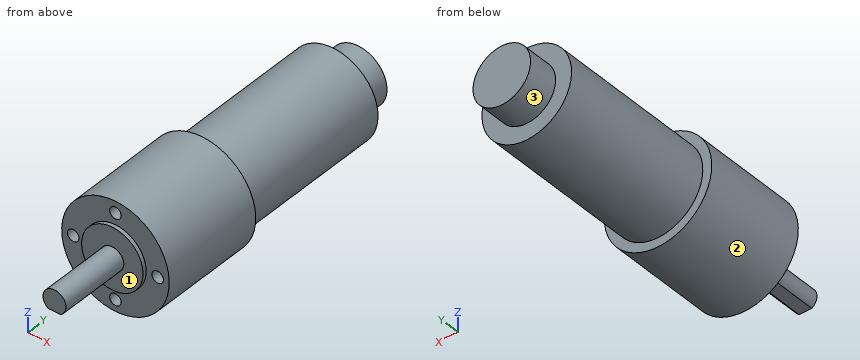
from build123d import *

# Parameters (mm, degrees)
SKETCH_1_R          = 14
EXTRUDE_1_DEPTH     = 27.7
SKETCH_3_R          = 11.669632126
EXTRUDE_2_DEPTH     = 42
SKETCH_8_R          = 7.5
EXTRUDE_4_DEPTH     = 8
SKETCH_9_R          = 8
EXTRUDE_5_DEPTH     = 1
SKETCH_5_R          = 3
EXTRUDE_3_DEPTH     = 18.5
CUT_EXTRUDE_START   = -12
CUT_EXTRUDE_2_DEPTH = 12
SKETCH_4_R          = 1.5
CUT_EXTRUDE_1_DEPTH = 4


with BuildPart() as part:
    # 草图1 → 凸台-拉伸1 (new body)
    with BuildSketch(Plane(origin=(0, 0, 0), x_dir=(1, 0, 0), z_dir=(0, 1, 0))):
        with Locations(Location((0, 0, 0), (0, 0, 270))):
            Circle(SKETCH_1_R)
    extrude(amount=EXTRUDE_1_DEPTH)

    # 草图3 → 凸台-拉伸2 (add)
    with BuildSketch(Plane(origin=(0, 27.7, 0), x_dir=(1, 0, 0), z_dir=(0, 1, 0))):
        with Locations(Location((0, 0, 0), (0, 0, 90))):
            Circle(SKETCH_3_R)
    extrude(amount=EXTRUDE_2_DEPTH)

    # 草图8 → 凸台-拉伸4 (add)
    with BuildSketch(Plane(origin=(0, 69.7, 0), x_dir=(1, 0, 0), z_dir=(0, 1, 0))):
        with Locations(Location((0, 0, 0), (0, 0, 270))):
            Circle(SKETCH_8_R)
    extrude(amount=EXTRUDE_4_DEPTH)

    # 草图9 → 凸台-拉伸5 (add)
    with BuildSketch(Plane.XZ):
        with Locations(Location((0, 0, 0), (0, 0, 90))):
            Circle(SKETCH_9_R)
    extrude(amount=EXTRUDE_5_DEPTH)

    # 草图5 → 凸台-拉伸3 (add)
    with BuildSketch(Plane.XZ.offset(1)):
        with Locations(Location((0, 0, 0), (0, 0, 270))):
            Circle(SKETCH_5_R)
    extrude(amount=EXTRUDE_3_DEPTH)

    # 草图7 → 切除-拉伸2 (cut)
    with BuildSketch(Plane.XZ.offset(19.5).offset(CUT_EXTRUDE_START)):
        with BuildLine():
            Line((-1.658312395, -2.5), (1.658312395, -2.5))
            ThreePointArc((1.658312395, -2.5), (0, -3), (-1.658312395, -2.5))
        make_face()
    extrude(amount=CUT_EXTRUDE_2_DEPTH, mode=Mode.SUBTRACT)

    # 草图4 → 切除-拉伸1 (cut)
    with BuildSketch(Plane.XZ):
        with Locations(Location((0, 11, 0), (0, 0, 270))):
            Circle(SKETCH_4_R)
        with Locations(Location((11, 0, 0), (0, 0, 270))):
            Circle(SKETCH_4_R)
        with Locations(Location((0, -11, 0), (0, 0, 270))):
            Circle(SKETCH_4_R)
        with Locations(Location((-11, 0, 0), (0, 0, 270))):
            Circle(SKETCH_4_R)
    extrude(amount=-CUT_EXTRUDE_1_DEPTH, mode=Mode.SUBTRACT)


solid = part.part
Verification items for the finished model (mm, model axes). Face numbers are marked on the shaded views. A direction names the side the tool comes from. Give positions to 0.01 mm unless a question says otherwise; leave off trailing zeros. Order: outer loops, then holes, each group sorted by start corner. A loop starts at its lowest first (then second) coordinate and runs counter-clockwise, first axis right, second up. Notation, with made-up numbers: (31, 26.25) -> (77, 26.25) arc R19 ccw to (77, 63.25) -> close; hole circle Ø11 at (78.25, 23). An arc over 180 degrees is marked (long way). Answer as CSV lines item,"result".
Q1. Sectioned sample at C-C on y = 15. Record the cut outline in (x, z).
Solutions:
outline,"circle Ø28 at (0, 0)"
Q2. Sectioned sample at A-A on z = 0. Record the cut outline in (x, y).
Solutions:
outline,"(-14, 0) -> (-12.5, 0) -> (-12.5, 4) -> (-9.5, 4) -> (-9.5, 0) -> (-8, 0) -> (-8, -1) -> (-3, -1) -> (-3, -19.5) -> (3, -19.5) -> (3, -1) -> (8, -1) -> (8, 0) -> (9.5, 0) -> (9.5, 4) -> (12.5, 4) -> (12.5, 0) -> (14, 0) -> (14, 27.7) -> (11.67, 27.7) -> (11.67, 69.7) -> (7.5, 69.7) -> (7.5, 77.7) -> (-7.5, 77.7) -> (-7.5, 69.7) -> (-11.67, 69.7) -> (-11.67, 27.7) -> (-14, 27.7) -> close"
Q3. Depth check by flat-ended pin: pin 1 (1.7 mm diameter, centred on x = -0.5, y = -14, fed in from -Z); pin 2 (2.5 mm diameter, centred on x = 10.5, z = 0.5, fed in from -Y); pin 3 (5 mm diameter, centred on y = 44, z = 10.5, fed in from +X). Enter the tip coordinate at first touch or a pass-through.
Solutions:
pin 1,"stops at z = -2.5"
pin 2,"stops at y = 0"
pin 3,"stops at x = 8.5"
Q4. Scan lines: probe 1 along X at (y, z) = (2.9, 0); probe 2 along X at (y, z) = (20, -0.25); probe 3 along X at (y, z) = (0.5, -12.25). Record each from-to range of solid material in increasing order.
Solutions:
probe 1,"x = -14 to -12.5, -9.5 to 9.5, 12.5 to 14"
probe 2,"x = -14 to 14"
probe 3,"x = -6.78 to -0.83, 0.83 to 6.78"
Q5. Access from +Z, -Z, +X, -X, +Y, -Y to the whole of each face (thin tool, end or side, straight path). Record for the marked faces 1, 2 and 3.
Solutions:
face 1,"-Y"
face 2,"+Y, -Y"
face 3,"+Y"
Q6. Sectioned sample at D-D on z = -4.75. Record the cut outline in (x, y), plus the area to 3 significant figures.
Solutions:
outline,"(-13.17, 0) -> (-6.44, 0) -> (-6.44, -1) -> (6.44, -1) -> (6.44, 0) -> (13.17, 0) -> (13.17, 27.7) -> (10.66, 27.7) -> (10.66, 69.7) -> (5.8, 69.7) -> (5.8, 77.7) -> (-5.8, 77.7) -> (-5.8, 69.7) -> (-10.66, 69.7) -> (-10.66, 27.7) -> (-13.17, 27.7) -> close"
area,"1,730 mm²"
